Autodesk Inventor part; units mm, degrees
ref_plane "YZ Plane" through (0, 0, 0) normal (1, 0, 0) x (0, 1, 0)
ref_plane "XZ Plane" through (0, 0, 0) normal (0, 1, 0) x (-1, 0, 0)
ref_plane "XY Plane" through (0, 0, 0) normal (0, 0, 1) x (1, 0, 0)
sketch "Sketch1" plane through (0, 0, 0) normal (0, 0, 1) x (1, 0, 0)
  line L0 (0, 0) -> (110, 0)
  line L1 (110, 0) -> (110, 10)
  line L2 (110, 10) -> (0, 10)
  line L3 (0, 10) -> (0, 0)
  circle A0 centre (10, 5) radius 1.6
  circle A1 centre (70, 5) radius 1.6
  circle A2 centre (105, 5) radius 1.6
  dimension "d0" = 110
  dimension "d1" = 10
  dimension "d2" = 90
  dimension "d3" = 110
  dimension "d4" = 3.2
  dimension "d6" = 3.2
  dimension "d7" = 3.2
  dimension "d8" = 60
  dimension "d9" = 35
extrude "Extrusion1" add sketch "Sketch1" along normal blind 11
sketch "Sketch2" plane through (0, 0, 0) normal (0, -1, 0) x (1, 0, 0)
  line L0 (0, 0) -> (0, 11)
  line L1 (110, 0) -> (110, 11)
  line L2 (0, 0) -> (110, 0)
  circle A0 centre (5, 7) radius 1.6
  circle A1 centre (75, 7) radius 1.6
  circle A2 centre (40, 7) radius 1.6
  dimension "d13" = 3.2
  dimension "d14" = 5
  dimension "d15" = 3.2
  dimension "d16" = 70
  dimension "d17" = 3.2
  dimension "d18" = 35
extrude "Extrusion2" cut sketch "Sketch2" against normal blind 10
sketch "Sketch3" plane through (0, 0, 11) normal (0, 0, 1) x (1, 0, 0)
  point P0 (0, 0)
sketch "Sketch4" plane through (0, 0, 11) normal (0, 0, 1) x (1, 0, 0)
  line L0 (13.4641, 5) -> (11.7321, 2)
  line L1 (11.7321, 2) -> (8.2679, 2)
  line L2 (8.2679, 2) -> (6.5359, 5)
  line L3 (6.5359, 5) -> (8.2679, 8)
  line L4 (8.2679, 8) -> (11.7321, 8)
  line L5 (11.7321, 8) -> (13.4641, 5)
  line L6 (73.4641, 5) -> (71.7321, 2)
  line L7 (71.7321, 2) -> (68.2679, 2)
  line L8 (68.2679, 2) -> (66.5359, 5)
  line L9 (66.5359, 5) -> (68.2679, 8)
  line L10 (68.2679, 8) -> (71.7321, 8)
  line L11 (71.7321, 8) -> (73.4641, 5)
  circle A0 centre (105, 5) radius 1.6
  line L12 (108.4641, 5) -> (106.7321, 2)
  line L13 (106.7321, 2) -> (103.2679, 2)
  line L14 (103.2679, 2) -> (101.5359, 5)
  line L15 (101.5359, 5) -> (103.2679, 8)
  line L16 (103.2679, 8) -> (106.7321, 8)
  line L17 (106.7321, 8) -> (108.4641, 5)
  point P0 (0, 0)
  point P1 (10, 5)
  point P2 (70, 5)
  dimension "d21" = 6
  dimension "d22" = 6
  dimension "d23" = 6
extrude "Extrusion3" cut sketch "Sketch4" against normal blind 3
properties part number "support"
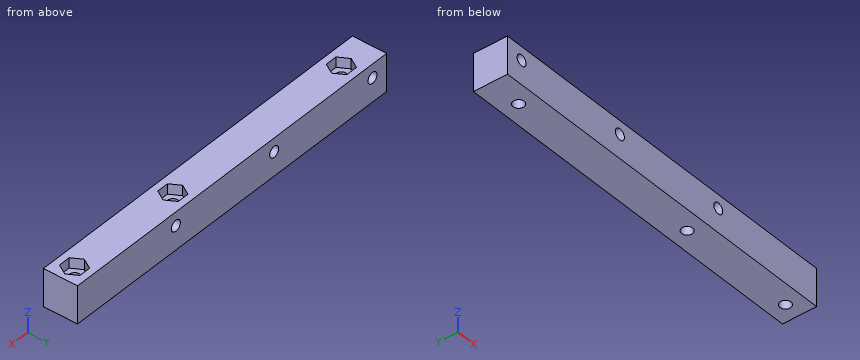
Could you check a few things on this model? Use its own coordinates, in mm. Round coordinates to 2 decimals unless told otherwise and drop trailing zeros. Order: outer loops, then holes, each group sorted by start corner. A loop starts at its lowest first (then second) coordinate and runs counter-clockwise, first axis right, second up. Notation, with made-up numbers: (39.25, 56.25) -> (85.25, 56.25) arc R28 cw to (85.25, 76.25) -> close; hole circle Ø8 at (35.5, 34.25). An arc over 180 degrees is marked (long way). One line per question, with ' | ' between items.
Q1. If we section it at C-C on z = 2.75: Write out the boundary of the cut face in (x, y), plus the area to 3 significant figures.
Computed values:
outline: (0, 0) -> (110, 0) -> (110, 10) -> (0, 10) -> close; hole circle Ø3.2 at (10, 5); hole circle Ø3.2 at (70, 5); hole circle Ø3.2 at (105, 5) | area: 1,080 mm²
Q2. If I drill on line 1 (Z direction, x = 40, y = 6.25); line 2 (X direction, y = 4.5, z = 3.75); line 3 (X direction, y = 4.75, z = 9.25), over which ranges is the centre line in solid material (lowest first)? Write a range as from..to.
Computed values:
line 1: 0..5.4, 8.6..11 | line 2: 0..8.48, 11.52..68.48, 71.52..103.48, 106.52..110 | line 3: 0..6.68, 13.32..66.68, 73.32..101.68, 108.32..110
Q3. If we section it at B-B on x = 10: Write out the boundary of the cut face in (y, z).
Computed values:
outline: (0, 0) -> (3.4, 0) -> (3.4, 8) -> (2, 8) -> (2, 11) -> (0, 11) -> close; (6.6, 0) -> (10, 0) -> (10, 11) -> (8, 11) -> (8, 8) -> (6.6, 8) -> close
Q4. If we section it at A-A on z = 7: Write out the boundary of the cut face in (x, y), plus the area to 3 significant figures.
Computed values:
outline: (0, 0) -> (3.4, 0) -> (3.4, 10) -> (0, 10) -> close; (6.6, 0) -> (38.4, 0) -> (38.4, 10) -> (6.6, 10) -> close; (41.6, 0) -> (73.4, 0) -> (73.4, 10) -> (41.6, 10) -> close; (76.6, 0) -> (110, 0) -> (110, 10) -> (76.6, 10) -> close; hole circle Ø3.2 at (10, 5); hole circle Ø3.2 at (70, 5); hole circle Ø3.2 at (105, 5) | area: 980 mm²
Q5. If we section it at D-D on x = 40: Write out the boundary of the cut face in (y, z).
Computed values:
outline: (0, 0) -> (10, 0) -> (10, 5.4) -> (0, 5.4) -> close; (0, 8.6) -> (10, 8.6) -> (10, 11) -> (0, 11) -> close
Q6. I'm going to push flat-ended pins straight in: pin 1 (3 mm diameter, centred on x = 105.5, y = 5, fed in from +Z); pin 2 (1.9 mm diameter, centred on x = 75, z = 7, fed in from -Y). Where does each tip first touch, or does it pass through?
Computed values:
pin 1: z = 8 | pin 2: through
